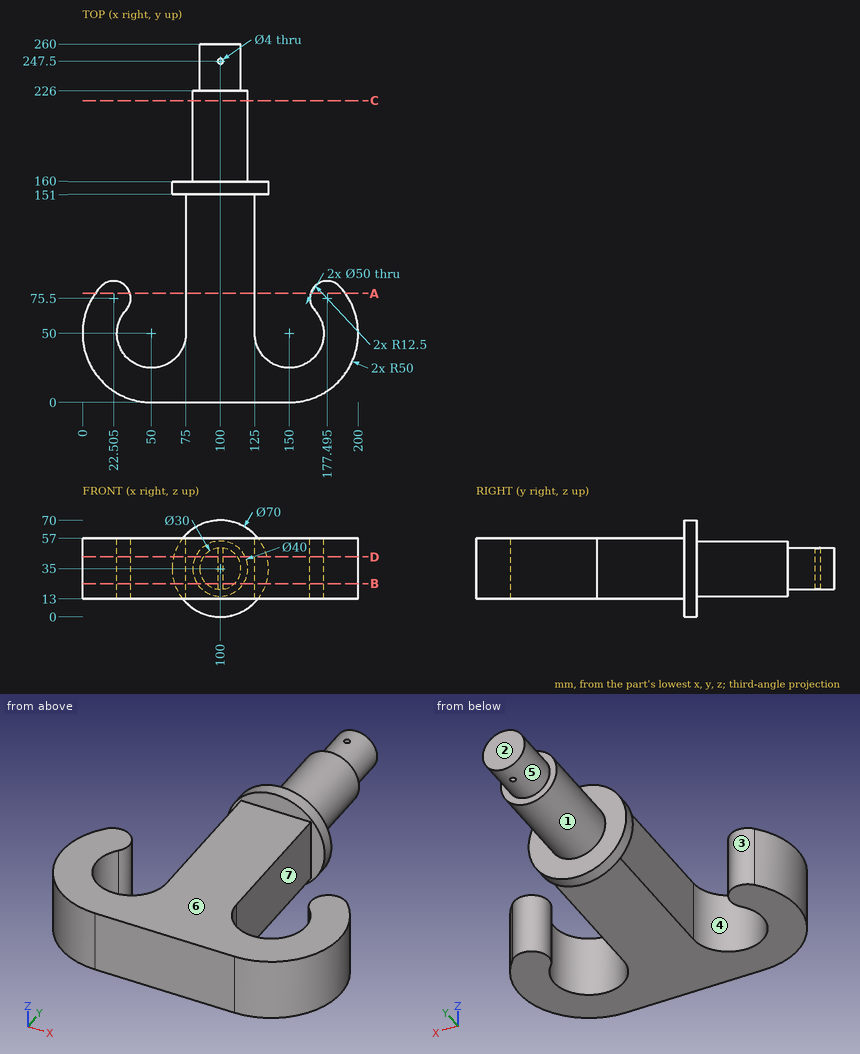
Answer from the drawing. Dimensions are ordinates in mm from the lowest x, y and z of the part. A direction names the side the tool comes from. Round coordinates to 2 decimals unless told otherwise and drop trailing zeros. Loops run counter-clockwise (first coordinate to the right, second up) from the corner with the lowest first, then second, coordinate; pieces in that order, holes last. Notation, with made-up numbers: M -35.75,43.25 L -4.75,43.25 A21 ccw -4.75,80.25 Z; hole C 8,85.25 d5. An arc over 180 degrees is marked long. One line per question, with ' | ' between items. Start each with the question number.
(1) For a pull along X with two mould halves and no side action, classify the marked faces 1, 2, 3 and 4 as released by +X, released by -X, zero draft, split by the parting line, or undercut.
(2) Find the intervals of material crossed by line 1 (X direction, y = 50, z = 31); line 2 (Y direction, x = 100, z = 38); line 3 (Z direction, x = 12, y = 18.5), in increasing order.
(3) A cutting plane is placed at B-B on z = 24. Write down the section's boundary in (x, y) (1 decimal).
(4) A cutting plane is placed at C-C on y = 219. Write down the section's boundary in (x, z).
(5) A cutting plane is placed at D-D on z = 43.5. Write down the section's boundary in (x, y) (1 decimal), plus the area to 3 significant figures.
(6) A cutting plane is placed at A-A on y = 79. Write down the section's boundary in (x, z) (1 decimal).
(7) A tool of negligible diameter and unlimited length cuts with its end or side. For the marked faces 5, 6 and 7, from which of +Z, -Z, +X, -X, +Y, -Y can it reach the whole face along a straight path? Write none if from no direction.
(8) Flat-ended cylindrical pins translate along their axes: pin 1 Ø1.5 at (y, z) = (92, 13) entering from -X; pin 2 Ø1.5 at (y, z) = (140, 51) entering from +X; pin 3 Ø4 at (x, y) = (173.5, 31.5) entering from -Z. Find the tip coordinate at first contact, or state that the pin passes through.
Geometry check:
1) face 1: split by the parting line | face 2: zero draft | face 3: undercut | face 4: undercut
2) line 1: x = 0 to 25, 75 to 125, 175 to 200 | line 2: y = 0 to 245.5, 249.5 to 260 | line 3: z = 13 to 57
3) outline: M 13.3,84 A50 ccw 50,0 L 150,0 A50 ccw 186.7,84 A12.5 ccw 168.3,67 A25 cw long 125,50 L 125,151 L 133.2,151 L 133.2,160 L 116.7,160 L 116.7,226 L 110.2,226 L 110.2,260 L 89.8,260 L 89.8,226 L 83.3,226 L 83.3,160 L 66.8,160 L 66.8,151 L 75,151 L 75,50 A25 cw long 31.7,67 A12.5 ccw Z; hole C 100,247.5 d4
4) outline: C 100,35 d40
5) outline: M 13.3,84 A50 ccw 50,0 L 150,0 A50 ccw 186.7,84 A12.5 ccw 168.3,67 A25 cw long 125,50 L 125,151 L 134,151 L 134,160 L 118.1,160 L 118.1,226 L 112.4,226 L 112.4,260 L 87.6,260 L 87.6,226 L 81.9,226 L 81.9,160 L 66,160 L 66,151 L 75,151 L 75,50 A25 cw long 31.7,67 A12.5 ccw Z; hole C 100,247.5 d4 | area: 17,700 mm²
6) outline: M 9.3,13 L 34.5,13 L 34.5,57 L 9.3,57 Z; M 75,13 L 125,13 L 125,57 L 75,57 Z; M 165.5,13 L 190.7,13 L 190.7,57 L 165.5,57 Z
7) face 5: +Y | face 6: +Z, +X, -X, -Y | face 7: +Z, -Z
8) pin 1: stops at x = 75 | pin 2: stops at x = 125 | pin 3: stops at z = 13
